For this review, use the dimensioned drawing (mm, ordinates from the lowest corner) and the shaded views. A direction names the side the tool comes from. Round coordinates to 2 decimals unless told otherwise and drop trailing zeros. Write each loop counter-clockwise with the first axis right and the second up, starting at its lowest first coordinate (ties: lowest second). Pieces come first, ordered by that corner, then holes. Notation, with made-up numbers: M 22.25,68.25 L 58.25,68.25 A18 cw 58.25,102.25 Z; hole C 11.5,87.25 d2. An arc over 180 degrees is marked long. One line per question, with ' | ' between items.
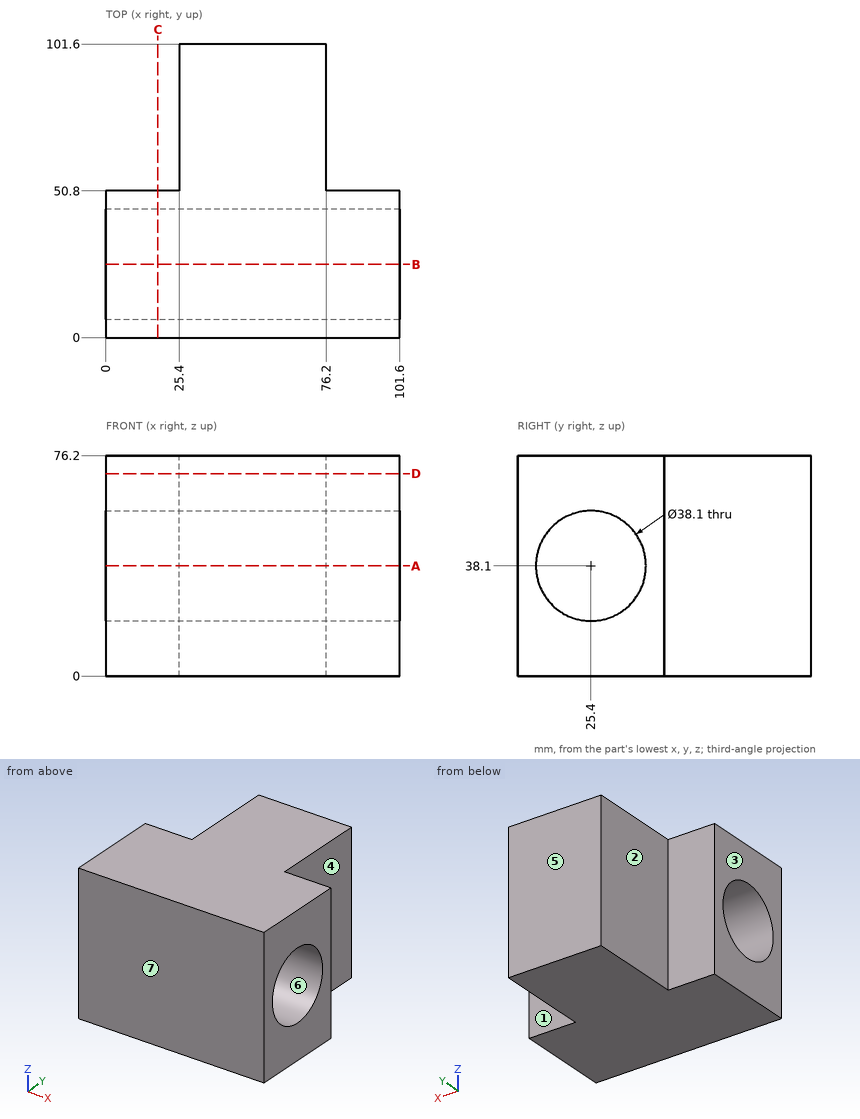
Item 1: Take a section at C-C (x = 18). Write out the cut boundary in (y, z), then the cut area to 3 significant figures.
Results:
outline: M 0,0 L 50.8,0 L 50.8,76.2 L 0,76.2 Z; hole C 25.4,38.1 d38.1 | area: 2,730 mm2
Item 2: Insertion check: pin 1 Ø20.5 at (x, z) = (8, 57) entering from +Y; pin 2 Ø1.5 at (y, z) = (90.5, 16) entering from -X. Each pin has a flat end and moves straight along its axis. Give the tip position at first contact, or say it passes through.
Results:
pin 1: y = 50.8 | pin 2: x = 25.4
Item 3: Take a section at A-A (z = 38.1). Write out the cut boundary in (x, y).
Results:
outline: M 0,0 L 101.6,0 L 101.6,6.35 L 0,6.35 Z; M 0,44.45 L 101.6,44.45 L 101.6,50.8 L 76.2,50.8 L 76.2,101.6 L 25.4,101.6 L 25.4,50.8 L 0,50.8 Z
Item 4: Take a section at B-B (y = 25.4). Write out the cut boundary in (x, z).
Results:
outline: M 0,0 L 101.6,0 L 101.6,19.05 L 0,19.05 Z; M 0,57.15 L 101.6,57.15 L 101.6,76.2 L 0,76.2 Z
Item 5: Mouldability with a two-part tool opening along Y and no side actions: class the marked faces 4, 5, 6 and 7 as +Y half, -Y half, draft (parallel to the pull), parting line (faces both ways), or undercut.
Results:
face 4: draft | face 5: +Y half | face 6: undercut | face 7: -Y half
Item 6: Machinability: for the marked faces 1, 2 and 3, which of the approach directions +Z, -Z, +X, -X, +Y, -Y give a long, thin tool a straight path to every point of the face, cutting with its end or side? Answer none if there is none.
Results:
face 1: +Z, -Z, +X, +Y | face 2: +Z, -Z, -X, +Y | face 3: +Z, -Z, -X, +Y, -Y
Item 7: To check wall thickness, follow line 1 along Z through (x, y) = (34, 25); line 2 along Y through (x, z) = (56, 38); line 3 along X through (y, z) = (75, 48). State the ranges of each line that lie inside material, in increasing order. Write a range as from..to.
Results:
line 1: 0..19.05, 57.15..76.2 | line 2: 0..6.35, 44.45..101.6 | line 3: 25.4..76.2
Item 8: Take a section at D-D (z = 70). Write out the cut boundary in (x, y), then the cut area to 3 significant figures.
Results:
outline: M 0,0 L 101.6,0 L 101.6,50.8 L 76.2,50.8 L 76.2,101.6 L 25.4,101.6 L 25.4,50.8 L 0,50.8 Z | area: 7,740 mm2
